Verification items for the finished model (mm, model axes). A direction names the side the tool comes from. Coordinates: 2 decimals unless noted, no trailing zeros. Loops run counter-clockwise (first coordinate to the right, second up) from the corner with the lowest first, then second, coordinate; pieces in that order, holes last. Notation, with made-up numbers: (68.5, 58) -> (88.5, 58) arc R18 cw to (88.5, 86) -> close; hole circle Ø4 at (13.5, 85). An arc over 180 degrees is marked (long way). Write item = value, one per line.
```python
from build123d import *

# Parameters (mm, degrees)
F1_DEPTH = 25.4


with BuildPart() as f1:
    # F0 (on Top) → F1 (new body)
    with BuildSketch(Plane.XY):
        with BuildLine():
            Line((0, 1.709418), (0, 0))
            Line((0, 0), (2.536132, 0))
            Line((2.536132, 0), (2.536132, 1.70942))
            Line((2.536132, 1.70942), (64.130943, 1.70942))
            Line((64.130943, 1.70942), (64.130943, 0))
            Line((64.130943, 0), (66.667075, 0))
            Line((66.667075, 0), (66.667075, 1.709418))
            ThreePointArc((66.667075, 1.709418), (65.063333, 3.541403), (64.130943, 5.790582))
            Line((64.130943, 5.790582), (2.536132, 5.790582))
            ThreePointArc((2.536132, 5.790582), (1.603742, 3.541403), (0, 1.709418))
        make_face()
    extrude(amount=F1_DEPTH)


solid = f1.part
```
1) Sectioned sample at A-A, the plane y = 0.8. Record the cut outline in (x, z), plus the area to 3 significant figures.
Ans:
outline = (0, 0) -> (2.54, 0) -> (2.54, 25.4) -> (0, 25.4) -> close; (64.13, 0) -> (66.67, 0) -> (66.67, 25.4) -> (64.13, 25.4) -> close
area = 129 mm2
2) Sectioned sample at C-C, the plane x = 29.5. Record the cut outline in (y, z), plus the area to 3 significant figures.
Ans:
outline = (1.71, 0) -> (5.79, 0) -> (5.79, 25.4) -> (1.71, 25.4) -> close
area = 104 mm2
3) Material ranges on line 1 (X direction, y = 0.4, z = 18.5); line 2 (Y direction, x = 14, z = 15.25); line 3 (X direction, y = 5.25, z = 10.25), recorded low to high.
Ans:
line_1 = 0 to 2.54, 64.13 to 66.67
line_2 = 1.71 to 5.79
line_3 = 2.39 to 64.28
4) Release check for a two-part mould opening along X. For faces 1 (the face through (0, 1, 13)), 2 (the face through (33, 4, 0)), 3 (the face through (64.131, 1, 13)) record: pulls with the +X half, pulls with the -X half, needs draft (parallel to the pull), parting line crosses it, or undercut.
Ans:
face_1 = pulls with the -X half
face_2 = needs draft
face_3 = undercut
5) Sectioned sample at D-D, the plane y = 4.95. Record the cut outline in (x, z).
Ans:
outline = (2.29, 0) -> (64.38, 0) -> (64.38, 25.4) -> (2.29, 25.4) -> close
6) Sectioned sample at B-B, the plane z = 17.25. Record the cut outline in (x, y), plus the area to 3 significant figures.
Ans:
outline = (0, 0) -> (2.54, 0) -> (2.54, 1.71) -> (64.13, 1.71) -> (64.13, 0) -> (66.67, 0) -> (66.67, 1.71) arc R7.5 cw to (64.13, 5.79) -> (2.54, 5.79) arc R7.5 cw to (0, 1.71) -> close
area = 268 mm2
7) Tool access check on faces 4 (the face through (33, 1.709, 13)), 5 (the face through (66.667, 1, 13)). Record the directions out of +Z, -Z, +X, -X, +Y, -Y that give a thin tool (end or side, any length) a straight path to the whole face; none if there is none.
Ans:
face_4 = +Z, -Z, -Y
face_5 = +Z, -Z, +X, +Y, -Y
8) Depth check by flat-ended pin: pin 1 Ø1 at (y, z) = (3, 3.5) entering from -X; pin 2 Ø12.5 at (x, z) = (30.5, 10) entering from -Y. Enter the tip coordinate at first touch or a pass-through.
Ans:
pin_1 = 0.82
pin_2 = 1.71
